Could you check a few things on this model? Use its own coordinates, in mm. A direction names the side the tool comes from. Round coordinates to 2 decimals unless told otherwise and drop trailing zeros. Loops run counter-clockwise (first coordinate to the right, second up) from the corner with the lowest first, then second, coordinate; pieces in that order, holes last. Notation, with made-up numbers: M 1.25,46.25 L 39.25,46.25 A20 ccw 39.25,72.25 Z; hole C -7,63 d1. An arc over 180 degrees is marked long. Answer in a Markdown table with one row per item.
```python
from build123d import *

# Parameters (mm, degrees)
BOSS_EXTRUDE1_DEPTH = 4
SKETCH4_R           = 4
SKETCH4_R_2         = 2
CUT_EXTRUDE1_DEPTH  = 1
BOSS_EXTRUDE2_DEPTH = 3
BOSS_EXTRUDE3_DEPTH = 2
SKETCH9_W           = 10.6
SKETCH9_H           = 4.6
CUT_EXTRUDE2_DEPTH  = 2


with BuildPart() as part:
    # Sketch1 → Boss-Extrude1 (new body)
    with BuildSketch(Plane.XY):
        Polygon((5.464935303, 12.361984253), (13.500030518, 1.254714966), (13.500030518, -1.495285034), (6.708221436, -1.495285034), (6.708221436, -2.495285034), (9.000030518, -2.495285034), (10.500030518, -3.495285034), (15.500030518, -3.495285034), (18.116729736, -12.435714722), (18.183807373, -12.766372681), (18.19442749, -13.103652954), (18.148162842, -13.43788147), (18.046356201, -13.759597778), (17.891937256, -14.059585571), (17.689239502, -14.329391479), (17.444122314, -14.561233521), (17.163482666, -14.74861145), (16.243865967, -15.159500122), (15.268463135, -15.410751343), (14.26473999, -15.495285034), (-14.26473999, -15.495285034), (-15.2684021, -15.410751343), (-16.243865967, -15.159500122), (-17.163482666, -14.74861145), (-17.444122314, -14.561233521), (-17.689239502, -14.329391479), (-17.891937256, -14.059585571), (-18.046356201, -13.759597778), (-18.148162842, -13.43788147), (-18.19442749, -13.103652954), (-18.183807373, -12.766372681), (-18.116729736, -12.435714722), (-15.499969482, -3.495285034), (-10.499969482, -3.495285034), (-8.999969482, -2.495285034), (-6.708221436, -2.495285034), (-6.708221436, -1.495285034), (-13.499969482, -1.495285034), (-13.499969482, 1.254714966), (-5.464935303, 12.361984253), (-4.947479248, 13.004714966), (-4.746734619, 13.221054077), (-3.915679932, 13.971450806), (-3.550689697, 14.243942261), (-2.715545654, 14.767288208), (-1.902435303, 15.142776489), (-1.102752686, 15.383102417), (-0.306915283, 15.495285034), (0.489349365, 15.480758667), (1.307891846, 15.333633423), (2.152435303, 15.041397095), (3.030548096, 14.586288452), (3.915679932, 13.971450806), (4.746795654, 13.221054077), (4.947479248, 13.004714966), align=None)
        Polygon((6.708221436, -10.495285034), (8.500030518, -10.495285034), (8.500030518, -5.495285034), (4.854156494, -5.495285034), (4.854156494, -8.995285034), (6.184661865, -8.995285034), (6.184661865, -9.495285034), (6.708221436, -9.495285034), align=None, mode=Mode.SUBTRACT)
        Polygon((-4.854095459, -5.495285034), (-8.499969482, -5.495285034), (-8.499969482, -10.495285034), (-6.708221436, -10.495285034), (-6.708221436, -9.495285034), (-6.184661865, -9.495285034), (-6.184661865, -8.995285034), (-4.854095459, -8.995285034), align=None, mode=Mode.SUBTRACT)
    extrude(amount=BOSS_EXTRUDE1_DEPTH)

    # Sketch4 → Cut-Extrude1 (cut)
    with BuildSketch(Plane.XY.offset(4)):
        with Locations((0, 8.442743212)):
            Circle(SKETCH4_R)
        with Locations((0, 8.442743212)):
            Circle(SKETCH4_R_2, mode=Mode.SUBTRACT)
    extrude(amount=-CUT_EXTRUDE1_DEPTH, mode=Mode.SUBTRACT)

    # Sketch7 → Boss-Extrude2 (add)
    with BuildSketch(Plane.XY.offset(4)):
        Polygon((-15.499969482, -3.495285034), (-18.116729736, -12.435714722), (-18.150268555, -12.601043701), (-18.183807373, -12.766372681), (-18.189117432, -12.935012817), (-18.19442749, -13.103652954), (-18.171295166, -13.270767212), (-18.148162842, -13.43788147), (-18.046356201, -13.759597778), (-17.891937256, -14.059585571), (-17.689239502, -14.329391479), (-17.444122314, -14.561233521), (-17.163482666, -14.74861145), (-16.243865967, -15.159500122), (-15.2684021, -15.410751343), (-14.26473999, -15.495285034), (14.26473999, -15.495285034), (15.268463135, -15.410751343), (16.243865967, -15.159500122), (17.163482666, -14.74861145), (17.444122314, -14.561233521), (17.689239502, -14.329391479), (17.891937256, -14.059585571), (18.046356201, -13.759597778), (18.148162842, -13.43788147), (18.19442749, -13.103652954), (18.183807373, -12.766372681), (15.500030518, -3.495285034), (10.500030518, -3.495285034), (9.000030518, -2.495285034), (6.708221436, -2.495285034), (-6.708221436, -2.495285034), (-8.999969482, -2.495285034), (-10.499969482, -3.495285034), align=None)
        Polygon((-8.499969482, -5.495285034), (-8.499969482, -10.495285034), (-6.708221436, -10.495285034), (-6.708221436, -9.495285034), (-6.184661865, -9.495285034), (-6.184661865, -8.995285034), (-4.854095459, -8.995285034), (-4.854095459, -5.495285034), align=None, mode=Mode.SUBTRACT)
        Polygon((4.854156494, -5.495285034), (8.500030518, -5.495285034), (8.500030518, -10.495285034), (6.708221436, -10.495285034), (6.708221436, -9.495285034), (6.184661865, -9.495285034), (6.184661865, -8.995285034), (4.854156494, -8.995285034), align=None, mode=Mode.SUBTRACT)
    extrude(amount=BOSS_EXTRUDE2_DEPTH)

    # Sketch8 → Boss-Extrude3 (add)
    with BuildSketch(Plane.XY.offset(7)):
        Polygon((-6.708221436, -2.495285034), (-8.999969482, -2.495285034), (-10.499969482, -3.495285034), (-10.499969482, -13.496460595), (10.500030518, -13.496460595), (10.500030518, -3.495285034), (9.000030518, -2.495285034), (6.708221436, -2.495285034), (4.854156494, -2.495285034), (4.854156494, -5.495285034), (8.500030518, -5.495285034), (8.500030518, -10.495285034), (6.708221436, -10.495285034), (-6.708221436, -10.495285034), (-8.499969482, -10.495285034), (-8.499969482, -5.495285034), (-4.854095459, -5.495285034), (-4.854095459, -2.495285034), align=None)
    extrude(amount=BOSS_EXTRUDE3_DEPTH)

    # Sketch9 → Cut-Extrude2 (cut)
    with BuildSketch(Plane(origin=(0, 0, 0), x_dir=(-1, 0, 0), z_dir=(0, 0, -1))):
        with Locations((0, 6.603957423)):
            Rectangle(SKETCH9_W, SKETCH9_H)
    extrude(amount=-CUT_EXTRUDE2_DEPTH, mode=Mode.SUBTRACT)


solid = part.part
```
1) I want a section at C-C, the plane y = 5. Please give me the cut outline in (x, z), plus the area to 3 significant figures.
Computed:
| item | result |
|---|---|
| outline | M -10.79,0 L -5.3,0 L -5.3,2 L 5.3,2 L 5.3,0 L 10.79,0 L 10.79,4 L 2.04,4 L 2.04,3 L -2.04,3 L -2.04,4 L -10.79,4 Z |
| area | 61.1 mm² |
2) Will these pins go through, and if not, where does the flat tip stop? P1, Ø4, axis at x = -4.5, z = 3, coming from the +Y side; P2, Ø1.2, axis at x = -0.5, y = 9, coming from the +Z side; P3, Ø1.5, axis at y = -9, z = 6.5, coming from the -X side; P4, Ø14.5, axis at x = -6, y = 2.5, coming from the +Z side.
Computed:
| item | result |
|---|---|
| P1 | stops at y = 14.87 |
| P2 | stops at z = 4 |
| P3 | stops at x = -17.33 |
| P4 | stops at z = 9 |
3) Which directions (+Z, -Z, +X, -X, +Y, -Y) give clear straight access to the entire face, cutting with the end or side of a thin tool? Please do faces 4 (the face through (-0.43, 6.49, 3.51)), 5 (the face through (-6.708, -2, 2)), 6 (the face through (-4.854, -4, 8)).
Computed:
| item | result |
|---|---|
| face 4 | +Z |
| face 5 | +Z, -Z, -X |
| face 6 | +Z, +Y |
4) I want a section at A-A, the plane x = 12.5. Please give me the cut outline in (y, z), plus the area to 3 significant figures.
Computed:
| item | result |
|---|---|
| outline | M -15.5,0 L -3.5,0 L -3.5,7 L -15.5,7 Z; M -1.5,0 L 2.64,0 L 2.64,4 L -1.5,4 Z |
| area | 101 mm² |
5) If we mould it in two halves opening along X, with no side actions, what happens to faces 1 (the face through (0, 7, 2)), 2 (the face through (-2.315, 14.952, 1.972)), 3 (the face through (15.7, -15.3, 3.5))? For each: released by +X, released by -X, zero draft, split by the parting line, or undercut.
Computed:
| item | result |
|---|---|
| face 1 | undercut |
| face 2 | released by -X |
| face 3 | released by +X |
6) I want a section at B-B, the plane z = 8. Please give me the cut outline in (x, y), plus the area to 3 significant figures.
Computed:
| item | result |
|---|---|
| outline | M -10.5,-13.5 L 10.5,-13.5 L 10.5,-3.5 L 9,-2.5 L 4.85,-2.5 L 4.85,-5.5 L 8.5,-5.5 L 8.5,-10.5 L -8.5,-10.5 L -8.5,-5.5 L -4.85,-5.5 L -4.85,-2.5 L -9,-2.5 L -10.5,-3.5 Z |
| area | 115 mm² |
7) I need wall thicknesses on line 1 (Y direction, x = 0, z = 3.7); line 2 (Y direction, x = -8, z = 5.25); line 3 (X direction, y = -0.5, z = 2). Which ranges of each line are inside material? Lowest first, please.
Computed:
| item | result |
|---|---|
| line 1 | y = -15.5 to 4.44, 6.44 to 10.44, 12.44 to 15.49 |
| line 2 | y = -15.5 to -10.5, -5.5 to -2.5 |
| line 3 | x = -13.5 to 13.5 |
8) I want a section at D-D, the plane z = 4.5. State how many separate pieces and enclosed holes the cut face has, plus the area to 3 significant figures.
Computed:
| item | result |
|---|---|
| separate pieces | 1 |
| enclosed holes | 2 |
| area | 396 mm² |
